from build123d import *

# Parameters (mm, degrees)
SKETCH1_W           = 4.675
SKETCH1_H           = 1
CUT_EXTRUDE1_DEPTH  = 5.675
CIRPATTERN1_COUNT   = 2
CIRPATTERN1_ANGLE   = 90
SKETCH5_R           = 0.4
BOSS_EXTRUDE1_DEPTH = 2.85


with BuildPart() as part:
    # Sketch1 → Revolve1 (revolve)
    with BuildSketch(Plane(origin=(0, 0, 0), x_dir=(0, 0, -1), z_dir=(1, 0, 0))):
        with Locations((2.3375, 19.5)):
            Rectangle(SKETCH1_W, SKETCH1_H)
    revolve(axis=Axis((0, 33.37320456, 0), (0, -1, 0)))

    # Sketch2 → Cut-Extrude1 (cut, symmetric)
    with BuildSketch(Plane(origin=(0, 0, 0), x_dir=(0, 0, -1), z_dir=(1, 0, 0))):
        with BuildLine():
            Line((-0.5, 20), (0.5, 20))
            ThreePointArc((0.5, 20), (0.321027237, 19.981039562), (0.15, 19.925))
            Line((0.15, 19.925), (0.15, 19.85))
            Line((0.15, 19.85), (-0.15, 19.85))
            Line((-0.15, 19.85), (-0.15, 19.925))
            ThreePointArc((-0.15, 19.925), (-0.321027237, 19.981039562), (-0.5, 20))
        make_face()
    cut_extrude1 = extrude(amount=CUT_EXTRUDE1_DEPTH, both=True, mode=Mode.SUBTRACT)

    # CirPattern1: Cut-Extrude1 ×2 about axis
    cirpattern1_axis = Axis((0, 33.37320456, 0), (0, 1, 0))
    for i in range(1, CIRPATTERN1_COUNT):
        add(cut_extrude1.rotate(cirpattern1_axis, i * CIRPATTERN1_ANGLE / (CIRPATTERN1_COUNT - 1)), mode=Mode.SUBTRACT)

    # Sketch1<3> → Revolve2 (revolve)
    with BuildSketch(Plane(origin=(0, 0, 0), x_dir=(0, 0, -1), z_dir=(1, 0, 0))):
        with BuildLine():
            Line((4.675, 20.15), (4.675, 20))
            Line((4.675, 20), (4.675, 19))
            Line((4.675, 19), (0, 19))
            Line((0, 19), (0, 0))
            Line((0, 0), (5.425, 0))
            Line((5.425, 0), (5.425, -0.15))
            Line((5.425, -0.15), (5.575, -0.15))
            ThreePointArc((5.575, -0.15), (6.282106781, 0.142893219), (6.575, 0.85))
            Line((6.575, 0.85), (6.575, 1.527924299))
            ThreePointArc((6.575, 1.527924299), (6.512072918, 1.957832927), (6.328571429, 2.351671028))
            ThreePointArc((6.328571429, 2.351671028), (6, 3.45), (6.328571429, 4.548328972))
            ThreePointArc((6.328571429, 4.548328972), (6.512072918, 4.942167073), (6.575, 5.372075701))
            Line((6.575, 5.372075701), (6.575, 19.15))
            ThreePointArc((6.575, 19.15), (6.282106781, 19.857106781), (5.575, 20.15))
            Line((5.575, 20.15), (4.675, 20.15))
        make_face()
    revolve(axis=Axis((0, 33.37320456, 0), (0, -1, 0)))

    # Sketch5 → Boss-Extrude1 (add)
    with BuildSketch(Plane.XZ):
        with Locations((0, 2.5)):
            Circle(SKETCH5_R)
        with Locations((0, -2.5)):
            Circle(SKETCH5_R)
    extrude(amount=BOSS_EXTRUDE1_DEPTH)


solid = part.part
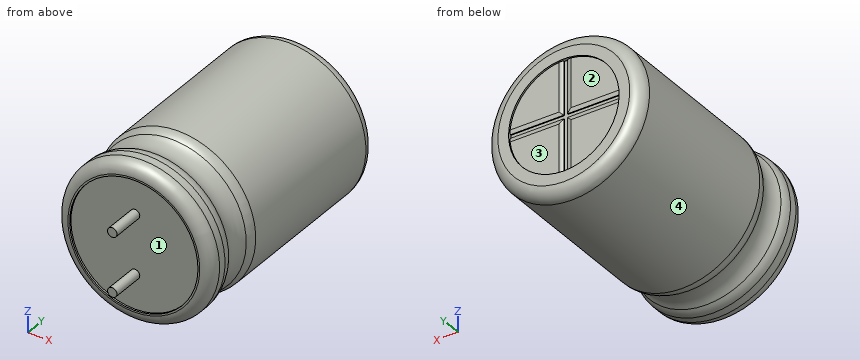
Design review of the part built by this model. Coordinates are the model's own, in mm. Face numbers are marked on the shaded views. A direction names the side the tool comes from. Coordinates: 2 decimals unless noted, no trailing zeros. Write each loop counter-clockwise with the first axis right and the second up, starting at its lowest first coordinate (ties: lowest second). Pieces come first, ordered by that corner, then holes. Notation, with made-up numbers: (79.25, 27) - (115.25, 27) arc R24 ccw to (115.25, 46) - close; hole circle Ø8 at (-7.5, 76). An arc over 180 degrees is marked (long way). Use one line per item in the form item = value.
Q1. Consider section C-C (y = 3.5). Write out the cut boundary in (x, z), plus the area to 3 significant figures.
Taken from the geometry:
outline = circle Ø12 at (0, 0)
area = 113 mm^2
Q2. The part is to be moulded in two halves that separate along Z. For the marked faces 3 and 4, say which applies: +Z half, -Z half, draft (parallel to the pull), parting line (faces both ways), or undercut.
Taken from the geometry:
face_3 = undercut
face_4 = parting line
Q3. For probe 1 along Y at (x, z) = (-0.25, 5); probe 2 along X at (y, z) = (19.9, 0) (3 decimals); probe 3 along Y at (x, z) = (4, 1.5), list the stretches that pass through material, from the lowest coordinate up.
Taken from the geometry:
probe_1 = 0 to 20.15
probe_2 = -6.236 to -4.675, 4.675 to 6.236
probe_3 = 0 to 20
Q4. Machinability: for the marked faces 1 and 2, which of the approach directions +Z, -Z, +X, -X, +Y, -Y give a long, thin tool a straight path to every point of the face, cutting with its end or side? Answer none if there is none.
Taken from the geometry:
face_1 = -Y
face_2 = +Y
Q5. Insertion check: pin 1 Ø3.5 at (x, z) = (-3, -2) entering from +Y; pin 2 Ø2 at (y, z) = (1, -2.5) entering from -X; pin 3 Ø2 at (y, z) = (15.5, -3) entering from +X; pin 4 Ø6.5 at (x, z) = (0, 0) entering from +Y. Each pin has a flat end and moves straight along its axis. Give the tip position at first contact, or say it passes through.
Taken from the geometry:
pin_1 = 20.15
pin_2 = -6.4
pin_3 = 6.26
pin_4 = 20
Q6. Consider section B-B (y = 11.5). Write out the cut boundary in (x, z) (3 decimals).
Taken from the geometry:
outline = circle Ø13.15 at (0, 0)
Q7. Consider section A-A (y = -1). Write out the cut boundary in (x, z).
Taken from the geometry:
outline = circle Ø0.8 at (0, -2.5); circle Ø0.8 at (0, 2.5)
